Verification items for the finished model (mm, model axes). Round coordinates to 2 decimals unless told otherwise and drop trailing zeros. Order: outer loops, then holes, each group sorted by start corner. A loop starts at its lowest first (then second) coordinate and runs counter-clockwise, first axis right, second up. Notation, with made-up numbers: (83, 4.5) -> (137, 4.5) arc R24 ccw to (137, 27.5) -> close; hole circle Ø1 at (17, 34.5). An arc over 180 degrees is marked (long way). Return JSON: item names as keys, results as strings. Group by question number.
1) Scan lines: L1, parallel to Y at x = 31.75, z = 0.3 (3 decimals); L2, parallel to Y at x = 41, z = 0.7. Record each from-to range of solid material in increasing order.
2) Section check D-D on x = 37. Enter the section's corners in (y, z), plus the area to 3 significant figures.
3) Section check C-C on z = 0.55. State how many separate pieces and enclosed holes the cut face has, plus the area to 3 significant figures.
4) Section check A-A on x = 44.45. Enter the section's corners in (y, z) (3 decimals), plus the area to 3 significant figures.
5) Section check B-B on y = 10.5. Enter the section's corners in (x, z).
6) Depth check by flat-ended pin: pin 1 (1.5 mm diameter, centred on x = 8.98, y = 6.89, fed in from +Z). Enter the tip coordinate at first touch or a pass-through.
7) Draft check along X on faces 1 (the cylindrical face through (47.62, 16.22, 0.39)), 2 (the flat face through (16, 16, 0.8)), 3 (the cylindrical face through (9.256, 26.095, 0.394)), 4 (the cylindrical face through (32.69, 27.72, 0.39)). Enter one of: pulls with the +X half, pulls with the -X half, needs draft (parallel to the pull), parting line crosses it, or undercut.
```python
from build123d import *

# Parameters (mm, degrees)
SKETCH1_R           = 3.2512
SKETCH1_R_2         = 1.27
BOSS_EXTRUDE1_DEPTH = 0.800000051
SKETCH3_R           = 0.4064
CUT_EXTRUDE3_DEPTH  = 58.243716905


with BuildPart() as part:
    # Sketch1 → Boss-Extrude1 (new body)
    with BuildSketch(Plane.XY):
        with BuildLine():
            Line((0, 31.75), (31.75, 31.75))
            ThreePointArc((31.75, 31.75), (47.625, 15.875), (31.75, 0))
            Line((31.75, 0), (0, 0))
            ThreePointArc((0, 0), (-15.875, 15.875), (0, 31.75))
        make_face()
        with Locations(Location((0, 15.875, 0), (0, 0, 180))):
            Circle(SKETCH1_R, mode=Mode.SUBTRACT)
        with Locations(Location((31.75, 15.875, 0), (0, 0, 180))):
            Circle(SKETCH1_R, mode=Mode.SUBTRACT)
        with Locations(Location((-12.7, 15.875, 0), (0, 0, 180))):
            Circle(SKETCH1_R_2, mode=Mode.SUBTRACT)
        with Locations(Location((-8.980256121, 24.855256121, 0), (0, 0, 180))):
            Circle(SKETCH1_R_2, mode=Mode.SUBTRACT)
        with Locations(Location((0, 28.575, 0), (0, 0, 180))):
            Circle(SKETCH1_R_2, mode=Mode.SUBTRACT)
        with Locations(Location((8.980256121, 24.855256121, 0), (0, 0, 180))):
            Circle(SKETCH1_R_2, mode=Mode.SUBTRACT)
        with Locations(Location((12.7, 15.875, 0), (0, 0, 180))):
            Circle(SKETCH1_R_2, mode=Mode.SUBTRACT)
        with Locations(Location((8.980256121, 6.894743879, 0), (0, 0, 180))):
            Circle(SKETCH1_R_2, mode=Mode.SUBTRACT)
        with Locations(Location((0, 3.175, 0), (0, 0, 180))):
            Circle(SKETCH1_R_2, mode=Mode.SUBTRACT)
        with Locations(Location((-8.980256121, 6.894743879, 0), (0, 0, 180))):
            Circle(SKETCH1_R_2, mode=Mode.SUBTRACT)
        with Locations(Location((31.75, 3.175, 0), (0, 0, 180))):
            Circle(SKETCH1_R_2, mode=Mode.SUBTRACT)
        with Locations(Location((40.730256121, 6.894743879, 0), (0, 0, 180))):
            Circle(SKETCH1_R_2, mode=Mode.SUBTRACT)
        with Locations(Location((22.769743879, 6.894743879, 0), (0, 0, 180))):
            Circle(SKETCH1_R_2, mode=Mode.SUBTRACT)
        with Locations(Location((19.05, 15.875, 0), (0, 0, 180))):
            Circle(SKETCH1_R_2, mode=Mode.SUBTRACT)
        with Locations(Location((22.769743879, 24.855256121, 0), (0, 0, 180))):
            Circle(SKETCH1_R_2, mode=Mode.SUBTRACT)
        with Locations(Location((31.75, 28.575, 0), (0, 0, 180))):
            Circle(SKETCH1_R_2, mode=Mode.SUBTRACT)
        with Locations(Location((40.730256121, 24.855256121, 0), (0, 0, 180))):
            Circle(SKETCH1_R_2, mode=Mode.SUBTRACT)
        with Locations(Location((44.45, 15.875, 0), (0, 0, 180))):
            Circle(SKETCH1_R_2, mode=Mode.SUBTRACT)
    extrude(amount=BOSS_EXTRUDE1_DEPTH)

    # Sketch3 → Cut-Extrude3 (cut, through all)
    with BuildSketch(Plane(origin=(0, 0, 0.800000051), x_dir=(-1, 0, 0), z_dir=(0, 0, -1))):
        with Locations((-14.605, 30.353)):
            Circle(SKETCH3_R)
        with Locations((-12.065, 30.353)):
            Circle(SKETCH3_R)
        with Locations((-9.525, 30.353)):
            Circle(SKETCH3_R)
        with Locations((-6.985, 30.353)):
            Circle(SKETCH3_R)
        with Locations(Location((-24.765, 30.353, 0), (0, 0, 180))):
            Circle(SKETCH3_R)
        with Locations(Location((-22.225, 30.353, 0), (0, 0, 180))):
            Circle(SKETCH3_R)
        with Locations(Location((-19.685, 30.353, 0), (0, 0, 180))):
            Circle(SKETCH3_R)
        with Locations(Location((-17.145, 30.353, 0), (0, 0, 180))):
            Circle(SKETCH3_R)
        with Locations((-17.145, 1.397)):
            Circle(SKETCH3_R)
        with Locations((-19.685, 1.397)):
            Circle(SKETCH3_R)
        with Locations((-22.225, 1.397)):
            Circle(SKETCH3_R)
        with Locations((-24.765, 1.397)):
            Circle(SKETCH3_R)
        with Locations(Location((-6.985, 1.397, 0), (0, 0, 180))):
            Circle(SKETCH3_R)
        with Locations(Location((-9.525, 1.397, 0), (0, 0, 180))):
            Circle(SKETCH3_R)
        with Locations(Location((-12.065, 1.397, 0), (0, 0, 180))):
            Circle(SKETCH3_R)
        with Locations(Location((-14.605, 1.397, 0), (0, 0, 180))):
            Circle(SKETCH3_R)
    extrude(amount=CUT_EXTRUDE3_DEPTH, mode=Mode.SUBTRACT)


solid = part.part
```
Check result:
{
 "1": {"L1": "0 to 1.905, 4.445 to 12.624, 19.126 to 27.305, 29.845 to 31.75", "L2": "2.97 to 5.65, 8.14 to 23.61, 26.1 to 28.78"},
 "2": {"outline": "(0.89, 0) -> (30.86, 0) -> (30.86, 0.8) -> (0.89, 0.8) -> close", "area": "24.0 mm^2"},
 "3": {"separate pieces": "1", "enclosed holes": "34", "area": "1,640 mm^2"},
 "4": {"outline": "(6.35, 0) -> (14.605, 0) -> (14.605, 0.8) -> (6.35, 0.8) -> close; (17.145, 0) -> (25.4, 0) -> (25.4, 0.8) -> (17.145, 0.8) -> close", "area": "13.2 mm^2"},
 "5": {"outline": "(-14.94, 0) -> (46.69, 0) -> (46.69, 0.8) -> (-14.94, 0.8) -> close"},
 "6": {"pin 1": "through"},
 "7": {"face 1": "pulls with the +X half", "face 2": "needs draft", "face 3": "undercut", "face 4": "undercut"}
}
